Autodesk Inventor part; units mm, degrees
ref_plane "YZ Plane" through (0, 0, 0) normal (1, 0, 0) x (0, 1, 0)
ref_plane "XZ Plane" through (0, 0, 0) normal (0, 1, 0) x (-1, 0, 0)
ref_plane "XY Plane" through (0, 0, 0) normal (0, 0, 1) x (1, 0, 0)
sketch "Sketch1" plane through (0, 0, 0) normal (0, 1, 0) x (-1, 0, 0)
  circle A0 centre (0, 0) radius 75
  line L0 (0, 0) -> (45.6571, 59.5015)
  line L1 (0, 0) -> (-45.6571, 59.5015)
  line L2 (0, 0) -> (0, 75)
  circle A1 centre (0, 0) radius 72.3
  circle A2 centre (0, 0) radius 91
  line L3 (45.6571, 59.5015) -> (45.6571, 56.06)
  line L4 (45.6571, 56.06) -> (60.6571, 56.06)
  line L5 (45.6571, 59.5015) -> (45.6571, 78.7174)
  line L6 (60.6571, 56.06) -> (60.6571, 61.06)
  line L7 (60.6571, 61.06) -> (45.6571, 61.06)
  line L8 (-45.6571, 59.5015) -> (-45.6571, 56.06)
  line L9 (-45.6571, 56.06) -> (-60.6571, 56.06)
  line L10 (-45.6571, 59.5015) -> (-45.6571, 78.7174)
  line L11 (-60.6571, 56.06) -> (-60.6571, 61.06)
  line L12 (-60.6571, 61.06) -> (-45.6571, 61.06)
  point P0 (44.0135, 57.3594)
  point P1 (-44.0135, 57.3594)
  dimension "d0" = 150
  dimension "d1" = 37.5
  dimension "d2" = 37.5
  dimension "d3" = 2.7
  dimension "d9" = 16
  dimension "d21" = 15
  dimension "d22" = 5
extrude "Extrusion1" add sketch "Sketch1" along normal blind 3 contours L5 L7 L6 L4 A0 | A0 L4 L3 | A0 L10 A2 L5 | L8 L9 A0 | A0 L9 L11 L12 L10
fillet "Fillet2" radius 5 2 edges at (-45.6571, 1.5, 78.7174) (45.6571, 1.5, 78.7174)
sketch "Sketch2" plane through (0, 3, 0) normal (0, 1, 0) x (1, 0, 0)
  circle A0 centre (-40.6571, -75.7826) radius 2
  circle A1 centre (40.6571, -75.7826) radius 2
  arc A2 (43.0209, -80.1885) -> (45.6571, -75.7826) centre (40.6571, -75.7826) ccw
  arc A3 (-45.6571, -75.7826) -> (-43.0209, -80.1885) centre (-40.6571, -75.7826) ccw
  point P0 (0, 0)
  dimension "d17" = 4
  dimension "d18" = 4
extrude "Extrusion2" cut sketch "Sketch2" against normal blind 3
fillet "Fillet5" radius 1 8 edges at (45.6571, 1.5, 56.06) (45.6571, 1.5, 59.5015) (60.6571, 1.5, 56.06) (60.6571, 1.5, 61.06) (-45.6571, 1.5, 56.06) (-45.6571, 1.5, 59.5015) (-60.6571, 1.5, 56.06) (-60.6571, 1.5, 61.06)
chamfer "Chamfer1" distance 8 angle 45 2 edges at (-45.6571, 1.5, 61.06) (45.6571, 1.5, 61.06)
fillet "Fillet7" radius 1 4 edges at (-53.6571, 1.5, 61.06) (-45.6571, 1.5, 69.06) (45.6571, 1.5, 69.06) (53.6571, 1.5, 61.06)
sketch "Sketch3" plane through (0, 3, 0) normal (0, 1, 0) x (1, 0, 0)
  arc A0 (-45.6571, -75.7826) -> (-43.0209, -80.1885) centre (-40.6571, -75.7826) ccw
  line L0 (-43.0209, -80.1885) -> (-28.0209, -80.1885)
  line L1 (-28.0209, -80.1885) -> (-28.0209, -95.1885)
  line L2 (-28.0209, -95.1885) -> (-43.0209, -95.1885)
  line L3 (-43.0209, -95.1885) -> (-43.0209, -80.1885)
  point P0 (0, 0)
  point P1 (-35.5209, -80.1885)
  dimension "d31" = 15
  dimension "d32" = 15
extrude "Extrusion3" add sketch "Sketch3" against normal blind 3
fillet "Fillet8" radius 1 3 edges at (-43.0209, 1.5, 80.1885) (-43.0209, 1.5, 95.1885) (-28.0209, 1.5, 95.1885)
fillet "Fillet9" radius 1 1 edges at (-28.0209, 1.5, 86.5785)
mirror "Mirror1" about plane through (0, 0, 0) normal (1, 0, 0) of "Extrusion3", "Fillet8", "Fillet9"
properties part number "Parte B bastantes piezas"
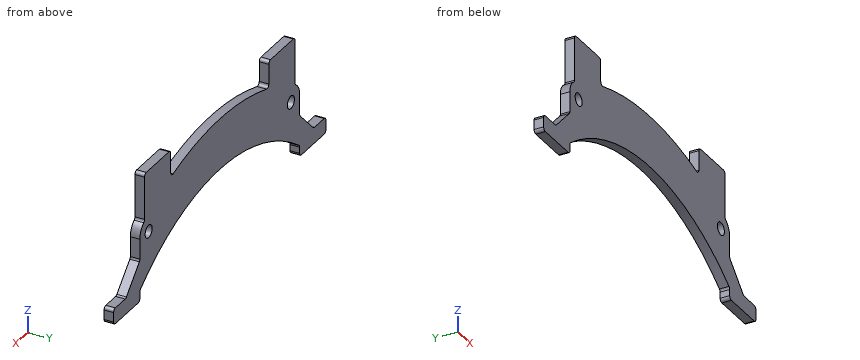
The listing builds one solid part. Answer for the finished solid, in the listing's coordinates (mm). Coordinates: 2 decimals unless noted, no trailing zeros. Write each loop counter-clockwise with the first axis right and the second up, starting at its lowest first coordinate (ties: lowest second). Pieces come first, ordered by that corner, then holes. Notation, with made-up numbers: (-9.75, 1) - (40.25, 1) arc R24 ccw to (40.25, 16) - close; hole circle Ø2 at (73, 13.5). An arc over 180 degrees is marked (long way). Return JSON: item names as keys, results as strings. Group by question number.
1. A cutting plane is placed at B-B, the plane x = -32.5. Determine the outline of the cut face in (y, z), plus the area to 3 significant figures.
2. Straight lines are drawn through the part: L1, parallel to X at y = 0.5, z = 92; L2, parallel to X at y = 1.7, z = 82.5; L3, parallel to X at y = 2, z = 63. For each, find the intervals that lie inside material, in ascending order.
3. A cutting plane is placed at C-C, the plane y = 1.45. Give the number of separate pieces and of enclosed holes in the cut face, plus the area to 3 significant figures.
4. Given pin 1 (0.9 mm diameter, centred on y = 1, z = 90, fed in from -X); pin 2 (1.5 mm diameter, centred on y = 1.5, z = 73, fed in from -X); pin 3 (1.5 mm diameter, centred on y = 1, z = 73, fed in from +X), each flat-ended and moving along its own axis, determine where each tip first touches the part or whether it passes through.
5. A cutting plane is placed at A-A, the plane z = 85. Determine the outline of the cut face in (x, y), plus the area to 3 significant figures.
Ans:
{
 "1": {"outline": "(0, 67.59) - (3, 67.59) - (3, 95.19) - (0, 95.19) - close", "area": "82.8 mm²"},
 "2": {"L1": "-43.02 to -28.02, 28.02 to 43.02", "L2": "-43.02 to 43.02", "L3": "-51.72 to -40.69, 40.69 to 51.72"},
 "3": {"separate pieces": "1", "enclosed holes": "2", "area": "2,080 mm²"},
 "4": {"pin 1": "x = -43.02", "pin 2": "x = -45.66", "pin 3": "x = 45.66"},
 "5": {"outline": "(-43.02, 0) - (43.02, 0) - (43.02, 3) - (-43.02, 3) - close", "area": "258 mm²"}
}
